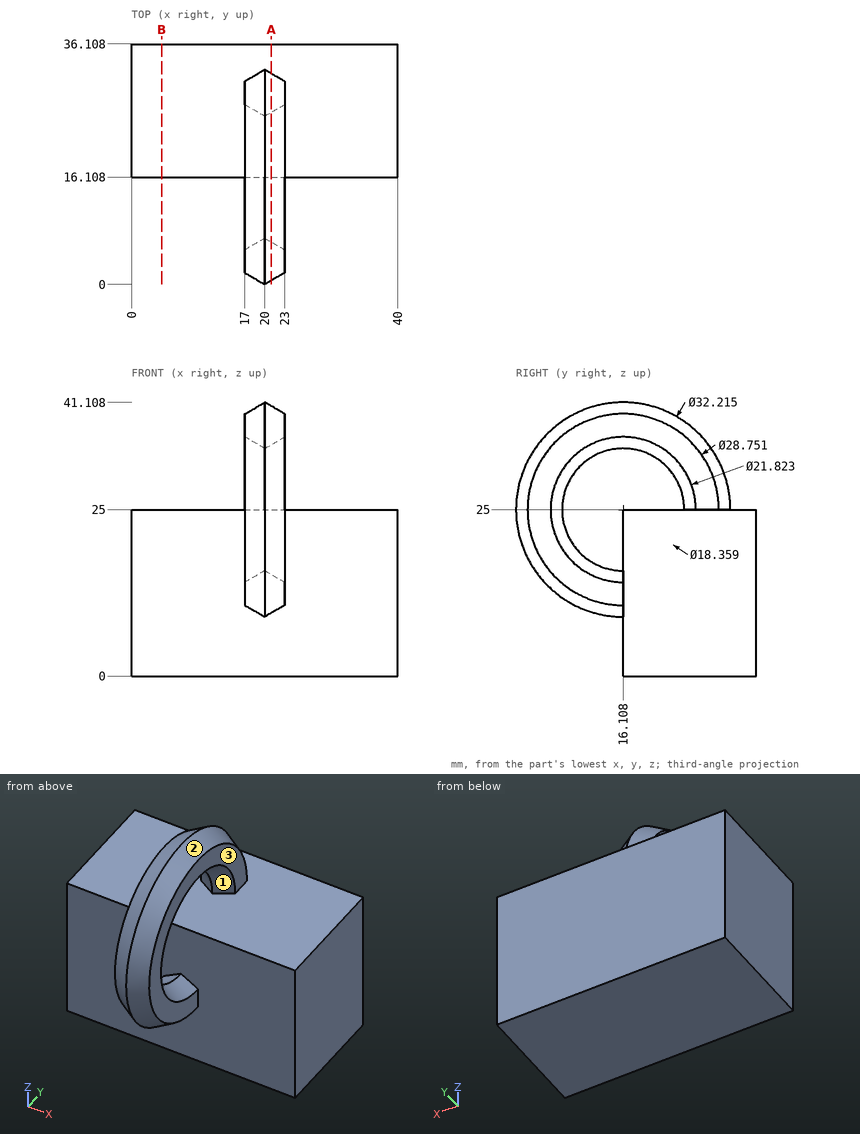
Answer from the drawing. Dimensions are ordinates in mm from the lowest x, y and z of the part. Give positions to 0.01 mm unless a question says otherwise; leave off trailing zeros. Order: outer loops, then holes, each group sorted by start corner. A loop starts at its lowest first (then second) coordinate and runs counter-clockwise, first axis right, second up. Notation, with made-up numbers: (48, 86) - (54, 86) arc R14 ccw to (54, 110) - close; hole circle Ø6 at (27.5, 57). An arc over 180 degrees is marked (long way). One line per item, written item: value. Start each with the question number.
1) A cutting plane is placed at A-A on x = 21. Give the vertices of the cut face in (y, z) (1 decimal), then the cut area to 3 significant figures.
2) The mould has two halves that part along Z. Classify the marked faces 1, 2 and 3: released by +Z, released by -Z, zero draft, split by the parting line, or undercut.
3) Find the intervals of material crossed by L1, parallel to Z at x = 5.5, y = 22; L2, parallel to X at y = 8, z = 33; L3, parallel to Y at x = 23, z = 7, in increasing order.
4) A cutting plane is placed at B-B on x = 4.5. Give the vertices of the cut face in (y, z), then the cut area to 3 significant figures.
5) Given pin 1 Ø4 at (x, y) = (16, 12.5) entering from -Z; pin 2 Ø8 at (x, z) = (5, 32.5) entering from -Y; pin 3 Ø3 at (x, z) = (13, 10.5) entering from -Y; pin 4 Ø1 at (y, z) = (31.5, 29.5) entering from +X, each flat-ended and moving along its own axis, determine where each tip first touches the part or whether it passes through.
Answer sheet:
1. outline: (16.1, 0) - (36.1, 0) - (36.1, 25) - (31.6, 25) arc R15.5 ccw (long way) to (16.1, 9.5) - close; hole (16.1, 15.2) - (16.1, 25) - (25.9, 25) arc R9.8 ccw (long way) to start
1. area: 844 mm2
2. face 1: undercut
2. face 2: split by the parting line
2. face 3: zero draft
3. L1: z = 0 to 25
3. L2: x = 17 to 23
3. L3: y = 16.11 to 36.11
4. outline: (16.11, 0) - (36.11, 0) - (36.11, 25) - (16.11, 25) - close
4. area: 500 mm2
5. pin 1: stops at z = 10.41
5. pin 2: passes through
5. pin 3: stops at y = 16.11
5. pin 4: stops at x = 20.99
